Autodesk Inventor part; units mm, degrees
ref_plane "NUT_XY" through (0, 0, 0) normal (0, 0, 1) x (1, 0, 0)
ref_plane "NUT_YZ" through (0, 0, 0) normal (1, 0, 0) x (0, 1, 0)
ref_plane "NUT_ZX" through (0, 0, 0) normal (0, 1, 0) x (0, 0, 1)
sketch "Sketch_8" plane through (0, 0, 0) normal (1, 0, 0) x (0, 1, 0)
  line L0 (0, -4.826) -> (0, 0)
  line L1 (0, 0) -> (6.35, 0)
  line L2 (6.35, 0) -> (7.62, -0.3403)
  line L3 (7.62, -0.3403) -> (7.62, -4.4857)
  line L4 (7.62, -4.4857) -> (6.35, -4.826)
  line L5 (6.35, -4.826) -> (0, -4.826)
  line L6 (0, -4.826) -> (0, 0)
sketch "Sketch_10" plane through (0, 0, 0) normal (0, 0, 1) x (1, 0, 0)
  line L0 (-12.7, -12.7) -> (12.7, -12.7)
  line L1 (12.7, -12.7) -> (12.7, 12.7)
  line L2 (12.7, 12.7) -> (-12.7, 12.7)
  line L3 (-12.7, 12.7) -> (-12.7, -12.7)
  line L4 (-6.35, -3.6662) -> (0, -7.3323)
  line L5 (0, -7.3323) -> (6.35, -3.6662)
  line L6 (6.35, -3.6662) -> (6.35, 3.6662)
  line L7 (6.35, 3.6662) -> (0, 7.3323)
  line L8 (0, 7.3323) -> (-6.35, 3.6662)
  line L9 (-6.35, 3.6662) -> (-6.35, -3.6662)
revolve "Revolution1" add sketch "Sketch_8" angle 360 about axis through (0, 0, -4.826) along (0, 0, -1)
extrude "Extrusion1" cut sketch "Sketch_10" against normal blind 4.826
sketch "Sketch_11" plane through (0, 0, 0) normal (1, 0, 0) x (0, 1, 0)
  line L0 (0, -4.826) -> (0, 0)
  line L1 (0, 0) -> (3.9688, 0)
  line L2 (3.9688, 0) -> (3.396, -0.5728)
  line L3 (3.396, -0.5728) -> (3.396, -4.2532)
  line L4 (3.396, -4.2532) -> (3.9688, -4.826)
  line L5 (3.9688, -4.826) -> (0, -4.826)
  line L6 (0, -4.826) -> (0, 0)
revolve "Revolution2" cut sketch "Sketch_11" angle 360 about axis through (0, 0, -4.826) along (0, 0, -1)
thread "Thread1"
ref_plane "NUT_XY" through (0, 0, 0) normal (0, 0, 1) x (1, 0, 0)
ref_plane "NUT_YZ" through (0, 0, 0) normal (1, 0, 0) x (0, 1, 0)
ref_plane "NUT_ZX" through (0, 0, 0) normal (0, 1, 0) x (0, 0, 1)
ref_plane "a1_XY" through (-6.35, 6.35, 0) normal (0, 0, 1) x (1, 0, 0)
ref_plane "a1_YZ" through (-6.35, 6.35, 0) normal (1, 0, 0) x (0, 1, 0)
ref_plane "a1_ZX" through (-6.35, 6.35, 0) normal (0, 1, 0) x (0, 0, 1)
ref_plane "a2_XY" through (6.35, 6.35, 0) normal (0, 0, 1) x (1, 0, 0)
ref_plane "a2_YZ" through (6.35, 6.35, 0) normal (1, 0, 0) x (0, 1, 0)
ref_plane "a2_ZX" through (6.35, 6.35, 0) normal (0, 1, 0) x (0, 0, 1)
ref_plane "b1_XY" through (0, 6.35, 0) normal (1, 0, 0) x (0, 0, -1)
ref_plane "b1_YZ" through (0, 6.35, 0) normal (0, 0, -1) x (0, 1, 0)
ref_plane "b1_ZX" through (0, 6.35, 0) normal (0, 1, 0) x (1, 0, 0)
ref_plane "b2_XY" through (0, 6.35, -4.826) normal (1, 0, 0) x (0, 0, -1)
ref_plane "b2_YZ" through (0, 6.35, -4.826) normal (0, 0, -1) x (0, 1, 0)
ref_plane "b2_ZX" through (0, 6.35, -4.826) normal (0, 1, 0) x (1, 0, 0)
ref_plane "e_XY" through (0, 0, -4.826) normal (1, 0, 0) x (0, 0, -1)
ref_plane "e_YZ" through (0, 0, -4.826) normal (0, 0, -1) x (0, 1, 0)
ref_plane "e_ZX" through (0, 0, -4.826) normal (0, 1, 0) x (1, 0, 0)
ref_plane "ol1_XY" through (0, 0, -6.35) normal (0, 1, 0) x (1, 0, 0)
ref_plane "ol1_YZ" through (0, 0, -6.35) normal (1, 0, 0) x (0, 0, -1)
ref_plane "ol1_ZX" through (0, 0, -6.35) normal (0, 0, -1) x (0, 1, 0)
ref_plane "ol2_XY" through (4.826, 0, -6.35) normal (0, 1, 0) x (1, 0, 0)
ref_plane "ol2_YZ" through (4.826, 0, -6.35) normal (1, 0, 0) x (0, 0, -1)
ref_plane "ol2_ZX" through (4.826, 0, -6.35) normal (0, 0, -1) x (0, 1, 0)
ref_plane "th1_XY" through (0, 3.9688, -4.826) normal (1, 0, 0) x (0, 0, -1)
ref_plane "th1_YZ" through (0, 3.9688, -4.826) normal (0, 0, -1) x (0, 1, 0)
ref_plane "th1_ZX" through (0, 3.9688, -4.826) normal (0, 1, 0) x (1, 0, 0)
ref_plane "th2_XY" through (0, -3.9688, -4.826) normal (1, 0, 0) x (0, 0, -1)
ref_plane "th2_YZ" through (0, -3.9688, -4.826) normal (0, 0, -1) x (0, 1, 0)
ref_plane "th2_ZX" through (0, -3.9688, -4.826) normal (0, 1, 0) x (1, 0, 0)
properties part number "D-746"
Verification items for the finished model (mm, model axes). Give positions to 0.01 mm unless a question says otherwise; leave off trailing zeros. Order: outer loops, then holes, each group sorted by start corner. A loop starts at its lowest first (then second) coordinate and runs counter-clockwise, first axis right, second up. Notation, with made-up numbers: M 44.5,30.5 L 50.5,30.5 A12 cw 50.5,48.5 Z; hole C 56.5,-23 d1. An arc over 180 degrees is marked long. Answer in a Markdown table with one row per item. Add a question column.
Item 1: Scan lines: probe 1 along X at (y, z) = (0, -2); probe 2 along X at (y, z) = (5.5, -4.2); probe 3 along Y at (x, z) = (3, -2.9). Record each from-to range of solid material in increasing order. Write a range as from..to.
Item 2: Gauge pin test, flat ends, axial feed: pin 1 (1.5 mm diameter, centred on x = 0, y = 3, fed in from -Z); pin 2 (2 mm diameter, centred on x = 2, y = -1, fed in from +Z). Record the tip position at first contact, or that the pin passes through.
Item 3: Mould release check, pull along X, two halves, no side actions. Record for faces 1 (the conical face through (-0.016, 6.589, -0.064)), 2 (the flat face through (-3, -3, 0)), 3 (the cylindrical face through (-2.07, -2.69, -2.44)): released by +X, released by -X, zero draft, split by the parting line, or undercut.
Item 4: Section check A-A, the plane z = -3.2. Enter the section's corners in (x, y), and give its area (3 significant figures).
Filled sheet:
| question | item | result |
|---|---|---|
| 1 | probe 1 | x = -6.35..-3.4, 3.4..6.35 |
| 1 | probe 2 | x = -3.17..3.17 |
| 1 | probe 3 | y = -5.6..-1.59, 1.59..5.6 |
| 2 | pin 1 | stops at z = -4.61 |
| 2 | pin 2 | passes through |
| 3 | face 1 | split by the parting line |
| 3 | face 2 | zero draft |
| 3 | face 3 | undercut |
| 4 | outline | M -6.35,-3.67 L 0,-7.33 L 6.35,-3.67 L 6.35,3.67 L 0,7.33 L -6.35,3.67 Z; hole C 0,0 d6.79 |
| 4 | area | 103 mm^2 |
